The drawing under review shows one solid part. Ordinate dimensions are in mm from its lowest x, y, z. A direction names the side the tool comes from. Coordinates: 2 decimals unless noted, no trailing zeros. Write each loop counter-clockwise with the first axis right and the second up, starting at its lowest first coordinate (ties: lowest second). Pieces come first, ordered by that corner, then holes. Notation, with made-up numbers: (32, 20) - (59, 20) arc R3 cw to (59, 25) - close; hole circle Ø10 at (-31.5, 7). An arc over 180 degrees is marked (long way). Put each result on its own line as item: value. Start each with the question number.
Item 1: Consider section C-C on z = 6.25. Give the boundary of the cut face in (x, y).
Item 2: Machinability: for the marked faces 4, 5, 6 and 7, which of the approach directions +Z, -Z, +X, -X, +Y, -Y give a long, thin tool a straight path to every point of the face, cutting with its end or side? Answer none if there is none.
Item 3: Consider section D-D on z = 3.75. Give the boundary of the cut face in (x, y), then the cut area to 3 significant figures.
Item 4: For pin 1 (13 mm diameter, centred on x = 17, y = 4.5, fed in from +Z); pin 2 (5.5 mm diameter, centred on x = 22.5, z = 6.5, fed in from +Y); pin 3 (3 mm diameter, centred on y = 19, z = 5, fed in from -X); pin 4 (1.2 mm diameter, centred on x = 25.5, z = 4, fed in from -Y), all flat-tipped, find the tip position at first contact; note any pin that passes through.
Item 5: Consider section B-B on y = 4. Give the boundary of the cut face in (x, z), then the cut area to 3 significant figures.
Item 6: Mouldability with a two-part tool opening along Y and no side actions: class the marked faces 1, 2 and 3 as pulls with the +Y half, pulls with the -Y half, needs draft (parallel to the pull), parting line crosses it, or undercut.
Item 7: Consider section A-A on x = 13. Give the boundary of the cut face in (y, z), then the cut area to 3 significant figures.
Item 8: To check wall thickness, follow L1, parallel to Y at x = 13, z = 3.95; L2, parallel to X at y = 4, z = 2.8; L3, parallel to Z at x = 22, y = 3.5. State the ranges of each line that lie inside material, in increasing order. Write a range as [from, to].
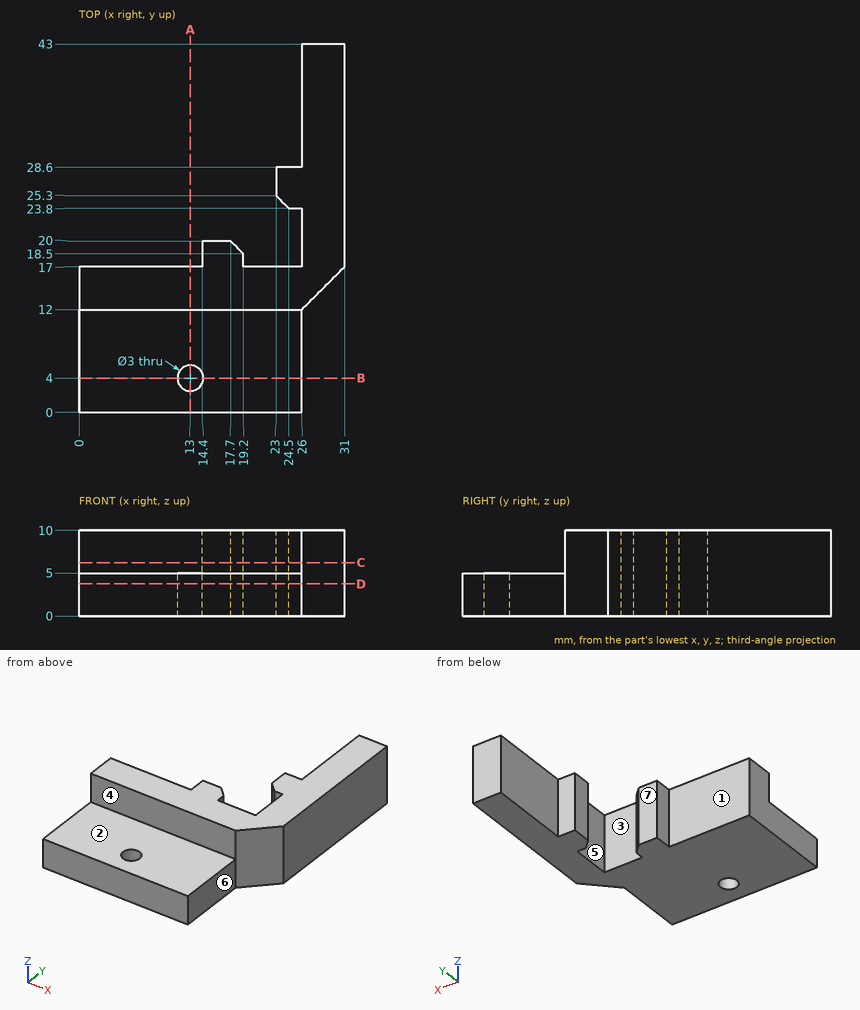
Report:
1. outline: (0, 12) - (26, 12) - (31, 17) - (31, 43) - (26, 43) - (26, 28.6) - (23, 28.6) - (23, 25.3) - (24.5, 23.8) - (26, 23.8) - (26, 17) - (19.2, 17) - (19.2, 18.5) - (17.7, 20) - (14.4, 20) - (14.4, 17) - (0, 17) - close
2. face 4: +Z, +X, -X, -Y
2. face 5: +Z, -Z
2. face 6: +Z, -Z, +X, -Y
2. face 7: +Z, -Z, -X, +Y
3. outline: (0, 0) - (26, 0) - (26, 12) - (31, 17) - (31, 43) - (26, 43) - (26, 28.6) - (23, 28.6) - (23, 25.3) - (24.5, 23.8) - (26, 23.8) - (26, 17) - (19.2, 17) - (19.2, 18.5) - (17.7, 20) - (14.4, 20) - (14.4, 17) - (0, 17) - close; hole circle Ø3 at (13, 4)
3. area: 604 mm²
4. pin 1: z = 5
4. pin 2: y = 28.6
4. pin 3: x = 14.4
4. pin 4: y = 0
5. outline: (0, 0) - (11.5, 0) - (11.5, 5) - (0, 5) - close; (14.5, 0) - (26, 0) - (26, 5) - (14.5, 5) - close
5. area: 115 mm²
6. face 1: pulls with the +Y half
6. face 2: needs draft
6. face 3: undercut
7. outline: (0, 0) - (2.5, 0) - (2.5, 5) - (0, 5) - close; (5.5, 0) - (17, 0) - (17, 10) - (12, 10) - (12, 5) - (5.5, 5) - close
7. area: 95.0 mm²
8. L1: [0, 2.5], [5.5, 17]
8. L2: [0, 11.5], [14.5, 26]
8. L3: [0, 5]
